```python
from build123d import *

# Parameters (mm, degrees)
F1_DEPTH = 5
F3_DEPTH = 40


with BuildPart() as f1:
    # F0 (on Top) → F1 (new body)
    with BuildSketch(Plane.XY):
        with BuildLine():
            ThreePointArc((0, 20), (5.857864, 5.857864), (20, 0))
            Line((20, 0), (150, 0))
            Line((150, 0), (150, 80))
            Line((150, 80), (80, 80))
            Line((80, 80), (80, 150))
            Line((80, 150), (0, 150))
            Line((0, 150), (0, 20))
        make_face()
    extrude(amount=F1_DEPTH)

    # F2 (on face) → F3 (join)
    with BuildSketch(Plane(origin=(0, 0, 0), x_dir=(1, 0, 0), z_dir=(0, 0, -1))):
        Polygon((80, -80), (150, -80), (150, -75), (75, -75), (75, -150), (80, -150), align=None)
    extrude(amount=F3_DEPTH)


solid = f1.part
```
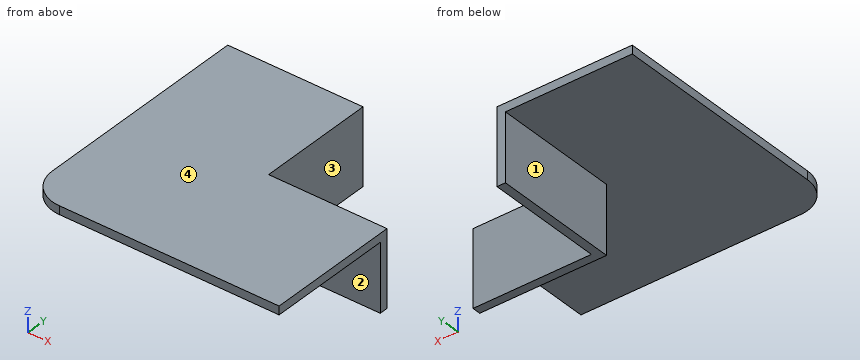
The model under review builds one solid part; all positions refer to its coordinate system, in mm. Face numbers are marked on the shaded views. A direction names the side the tool comes from. Round coordinates to 2 decimals unless told otherwise and drop trailing zeros. Loops run counter-clockwise (first coordinate to the right, second up) from the corner with the lowest first, then second, coordinate; pieces in that order, holes last. Notation, with made-up numbers: (78.5, -12.75) - (110.5, -12.75) arc R20 ccw to (110.5, 12.25) - close; hole circle Ø6 at (39.5, -33). An arc over 180 degrees is marked (long way). Use a Markdown table: item, result. Add a question column.
Q1. For probe 1 along Z at (x, y) = (24, 54.5); probe 2 along X at (y, z) = (89.5, -13), list the stretches that pass through material, from the lowest coordinate up.
Q2. Insertion check: pin 1 Ø1 at (x, y) = (31.5, 112.5) entering from -Z; pin 2 Ø12 at (x, z) = (119.5, -12.5) entering from -Y; pin 3 Ø10 at (y, z) = (99.5, -0.5) entering from +X. Each pin has a flat end and moves straight along its axis. Give the tip position at first contact, or say it passes through.
Q3. Add section A-A (y = 78). State the section outline as (x, z) points.
Q4. Machinability: for the marked faces 1, 2, 3 and 4, which of the approach directions +Z, -Z, +X, -X, +Y, -Y give a long, thin tool a straight path to every point of the face, cutting with its end or side? Answer none if there is none.
Q5. Add section C-C (y = 25). State the section outline as (x, z) points, plus the area to 3 significant figures.
Q6. Add section B-B (x = 122.5). State the section outline as (y, z) points, plus the area to 3 significant figures.
Worked answers:
| question | item | result |
|---|---|---|
| 1 | probe 1 | 0 to 5 |
| 1 | probe 2 | 75 to 80 |
| 2 | pin 1 | z = 0 |
| 2 | pin 2 | y = 75 |
| 2 | pin 3 | x = 80 |
| 3 | outline | (0, 0) - (75, 0) - (75, -40) - (150, -40) - (150, 5) - (0, 5) - close |
| 4 | face 1 | -Z, -X, +Y, -Y |
| 4 | face 2 | -Z, +X, -X, -Y |
| 4 | face 3 | +Z, -Z, +X, +Y |
| 4 | face 4 | +Z, +X, -X, +Y, -Y |
| 5 | outline | (0, 0) - (150, 0) - (150, 5) - (0, 5) - close |
| 5 | area | 750 mm² |
| 6 | outline | (0, 0) - (75, 0) - (75, -40) - (80, -40) - (80, 5) - (0, 5) - close |
| 6 | area | 600 mm² |
